The listing builds one solid part. Answer for the finished solid, in the listing's coordinates (mm). A direction names the side the tool comes from. Round coordinates to 2 decimals unless told otherwise and drop trailing zeros. Write each loop counter-clockwise with the first axis right and the second up, starting at its lowest first coordinate (ties: lowest second). Pieces come first, ordered by that corner, then holes.
(1) A cutting plane is placed at A-A, the plane y = 0. Give the vertices of the cut face in (x, z).
(2) A cutting plane is placed at B-B, the plane y = 4. Give the vertices of the cut face in (x, z), and give its area (3 significant figures).
(3) Find the intervals of material crossed by probe 1 along Y at (x, z) = (0, 1.7); probe 2 along X at (y, z) = (0, 15.15); probe 3 along Z at (x, y) = (3.75, -2), in increasing order.
(4) The mould has two halves that part along X. Classify faces 4 (the face through (0, 10.4, 9)), 5 (the face through (9, 10.4, 2)), 6 (the face through (-7.544, 12.865, -7.931)): +X half, -X half, draft (parallel to the pull), parting line (faces both ways), or undercut.
(5) For faces 1 (the face through (-5.04, -6, 16)), 2 (the face through (0, -6, 18)), 3 (the face through (-5.637, 12.865, 32.8)), determine the directions among +Z, -Z, +X, -X, +Y, -Y from which every point of the face is accessible in a straight line to the end or side of a thin tool.
(6) A cutting plane is placed at C-C, the plane z = 8.5. Give the vertices of the cut face in (x, y), and give its area (3 significant figures).
(7) Each of these flat-tipped pins is pushed along its axis until it touches: pin 1 Ø3 at (x, y) = (1.5, -8) entering from -Z; pin 2 Ø14.5 at (x, z) = (0, 9.01) entering from +Y; pin 3 Ø10 at (x, y) = (5.5, 0) entering from +Z. Where does it stop, or does it pass through?
(8) A cutting plane is placed at D-D, the plane z = -17. Give the vertices of the cut face in (x, y), and give its area (3 significant figures).
from build123d import *

# Parameters (mm, degrees)
CROQUIS1_W                 = 10.074318824
CROQUIS1_H                 = 23.311592876
CROQUIS1_R                 = 1.513350195
CROQUIS1_R_2               = 1.5
SALIENTE_EXTRUIR1_DEPTH    = 18
CROQUIS2_W                 = 10.074318824
CROQUIS2_H                 = 18
SALIENTE_EXTRUIR2_DEPTH    = 5
CORTAR_EXTRUIR1_DEPTH      = 22
SALIENTE_EXTRUIR3_DEPTH    = 5
CROQUIS5_R                 = 10
CROQUIS5_R_2               = 8
SALIENTE_EXTRUIR4_DEPTH    = 5
CORTAR_EXTRUIR3_DEPTH      = 33
CORTAR_EXTRUIR3_DEPTH_BACK = 14
CROQUIS7_R                 = 1.475964283
CROQUIS11_R                = 8.5
CROQUIS11_R_2              = 6.35
SALIENTE_EXTRUIR6_DEPTH    = 5
CROQUIS12_R                = 8.5
CROQUIS12_R_2              = 6.35
SALIENTE_EXTRUIR8_DEPTH    = 5
CORTAR_EXTRUIR4_DEPTH      = 22
CORTAR_EXTRUIR4_DEPTH_BACK = 14
CROQUIS13_R                = 1.510922734
CORTAR_EXTRUIR5_DEPTH      = 25
CORTAR_EXTRUIR5_DEPTH_BACK = 24
CROQUIS14_R                = 1.5177653


with BuildPart() as part:
    # Croquis1 → Saliente-Extruir1 (new body)
    with BuildSketch(Plane.XY):
        with Locations((-0.003103843, -6.255796438)):
            Rectangle(CROQUIS1_W, CROQUIS1_H)
        Circle(CROQUIS1_R, mode=Mode.SUBTRACT)
        with Locations((0, -12.5)):
            Circle(CROQUIS1_R_2, mode=Mode.SUBTRACT)
    extrude(amount=SALIENTE_EXTRUIR1_DEPTH)

    # Croquis2 → Saliente-Extruir2 (add)
    with BuildSketch(Plane(origin=(0, 5.4, 0), x_dir=(1, 0, 0), z_dir=(0, 1, 0))):
        with Locations((-0.003103843, -9)):
            Rectangle(CROQUIS2_W, CROQUIS2_H)
    extrude(amount=SALIENTE_EXTRUIR2_DEPTH)

    # Croquis3 → Cortar-Extruir1 (cut)
    with BuildSketch(Plane(origin=(5.034055569, 0, 0), x_dir=(0, 0, -1), z_dir=(1, 0, 0))):
        Polygon((-9, -17.911592876), (-13.015052671, -17.911592876), (-13.015052671, 5.408457803), (-4.97666887, 5.408457803), (-4.97666887, -17.911592876), align=None)
    extrude(amount=-CORTAR_EXTRUIR1_DEPTH, mode=Mode.SUBTRACT)

    # Croquis4 → Saliente-Extruir3 (add)
    with BuildSketch(Plane(origin=(0, 10.4, 0), x_dir=(1, 0, 0), z_dir=(0, 1, 0))):
        Polygon((-0.003103843, 22.715254114), (12.996896157, 22.715254114), (12.996896157, -40.731801261), (-13.003103843, -40.731801261), (-13.003103843, 22.715254114), align=None)
    extrude(amount=-SALIENTE_EXTRUIR3_DEPTH)

    # Croquis5 → Saliente-Extruir4 (add)
    with BuildSketch(Plane(origin=(0, 10.4, 0), x_dir=(1, 0, 0), z_dir=(0, 1, 0))):
        with Locations(Location((-0.003103843, -9.008273573, 0), (0, 0, 270))):
            Circle(CROQUIS5_R)
        with Locations(Location((-0.003103843, -9.008273573, 0), (0, 0, 270))):
            Circle(CROQUIS5_R_2, mode=Mode.SUBTRACT)
    extrude(amount=SALIENTE_EXTRUIR4_DEPTH)

    # Croquis7 → Cortar-Extruir3 (cut, two sides: drawn at the far end of the back side and taken through both)
    with BuildSketch(Plane(origin=(0, 0, 0), x_dir=(0, 0, -1), z_dir=(1, 0, 0)).offset(-CORTAR_EXTRUIR3_DEPTH_BACK)):
        with Locations(Location((-9.008273573, 12.900838069, 0), (0, 0, 180))):
            Circle(CROQUIS7_R)
    extrude(amount=CORTAR_EXTRUIR3_DEPTH + CORTAR_EXTRUIR3_DEPTH_BACK, mode=Mode.SUBTRACT)

    # Croquis11 → Saliente-Extruir6 (add)
    with BuildSketch(Plane(origin=(0, 10.4, 0), x_dir=(1, 0, 0), z_dir=(0, 1, 0))):
        with Locations(Location((-0.003103843, 11.85349027, 0), (0, 0, 270))):
            Circle(CROQUIS11_R)
        with Locations(Location((-0.003103843, 11.85349027, 0), (0, 0, 270))):
            Circle(CROQUIS11_R_2, mode=Mode.SUBTRACT)
    extrude(amount=SALIENTE_EXTRUIR6_DEPTH)

    # Croquis12 → Saliente-Extruir8 (add)
    with BuildSketch(Plane(origin=(0, 10.4, 0), x_dir=(1, 0, 0), z_dir=(0, 1, 0))):
        with Locations(Location((-0.003103843, -29.870037417, 0), (0, 0, 270))):
            Circle(CROQUIS12_R)
        with Locations(Location((-0.003103843, -29.870037417, 0), (0, 0, 270))):
            Circle(CROQUIS12_R_2, mode=Mode.SUBTRACT)
    extrude(amount=SALIENTE_EXTRUIR8_DEPTH)

    # Croquis13 → Cortar-Extruir4 (cut, two sides: drawn at the far end of the back side and taken through both)
    with BuildSketch(Plane(origin=(0, 0, 0), x_dir=(0, 0, -1), z_dir=(1, 0, 0)).offset(-CORTAR_EXTRUIR4_DEPTH_BACK)):
        with Locations(Location((11.85349027, 12.8884556, 0), (0, 0, 180))):
            Circle(CROQUIS13_R)
    extrude(amount=CORTAR_EXTRUIR4_DEPTH + CORTAR_EXTRUIR4_DEPTH_BACK, mode=Mode.SUBTRACT)

    # Croquis14 → Cortar-Extruir5 (cut, two sides: drawn at the far end of the back side and taken through both)
    with BuildSketch(Plane(origin=(0, 0, 0), x_dir=(0, 0, -1), z_dir=(1, 0, 0)).offset(-CORTAR_EXTRUIR5_DEPTH_BACK)):
        with Locations(Location((-29.870037417, 12.963711877, 0), (0, 0, 180))):
            Circle(CROQUIS14_R)
    extrude(amount=CORTAR_EXTRUIR5_DEPTH + CORTAR_EXTRUIR5_DEPTH_BACK, mode=Mode.SUBTRACT)


solid = part.part
Solutions:
1. outline: (-5.04, 0) - (-1.51, 0) - (-1.51, 4.98) - (-5.04, 4.98) - close; (-5.04, 13.02) - (-1.51, 13.02) - (-1.51, 18) - (-5.04, 18) - close; (1.51, 0) - (5.03, 0) - (5.03, 4.98) - (1.51, 4.98) - close; (1.51, 13.02) - (5.03, 13.02) - (5.03, 18) - (1.51, 18) - close
2. outline: (-5.04, 0) - (5.03, 0) - (5.03, 4.98) - (-5.04, 4.98) - close; (-5.04, 13.02) - (5.03, 13.02) - (5.03, 18) - (-5.04, 18) - close
2. area: 100 mm2
3. probe 1: y = -17.91 to -14, -11 to -1.51, 1.51 to 10.4
3. probe 2: x = -5.04 to -1.51, 1.51 to 5.03
3. probe 3: z = 0 to 4.98, 13.02 to 18
4. face 4: undercut
4. face 5: draft
4. face 6: parting line
5. face 1: +Z, -Z, -X, -Y
5. face 2: +Z, +X, -X, -Y
5. face 3: +Y
6. outline: (-13, 5.4) - (13, 5.4) - (13, 10.4) - (9.98, 10.4) - (9.98, 11.52) - (7.98, 11.52) - (7.98, 10.4) - (-7.99, 10.4) - (-7.99, 11.52) - (-9.99, 11.52) - (-9.99, 10.4) - (-13, 10.4) - close; (-9.99, 14.29) - (-7.99, 14.29) - (-7.99, 15.4) - (-9.99, 15.4) - close; (7.98, 14.29) - (9.98, 14.29) - (9.98, 15.4) - (7.98, 15.4) - close
6. area: 139 mm2
7. pin 1: stops at z = 0
7. pin 2: stops at y = 10.4
7. pin 3: stops at z = 18
8. outline: (-13, 5.4) - (13, 5.4) - (13, 10.4) - (6.76, 10.4) - (6.76, 15.4) - (3.72, 15.4) - (3.72, 10.4) - (-3.72, 10.4) - (-3.72, 15.4) - (-6.77, 15.4) - (-6.77, 10.4) - (-13, 10.4) - close
8. area: 160 mm2
